Answer from the drawing. Dimensions are ordinates in mm from the lowest x, y and z of the part. Give positions to 0.01 mm unless a question says otherwise; leave off trailing zeros. Loops run counter-clockwise (first coordinate to the right, second up) from the corner with the lowest first, then second, coordinate; pieces in that order, holes last. Notation, with made-up numbers: (7, 40.25) -> (54, 40.25) arc R32 cw to (54, 72.25) -> close; hole circle Ø7 at (-38.5, 77.5). An arc over 180 degrees is marked (long way). Answer as CSV lines item,"result". Start each with the question number.
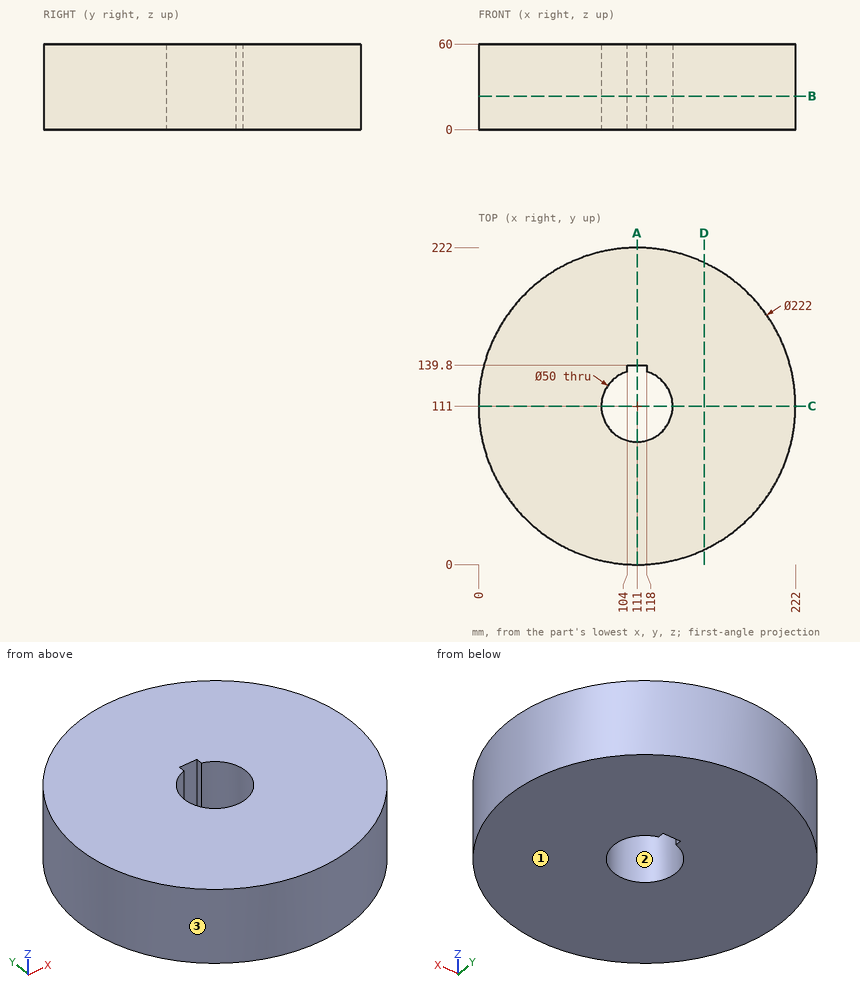
(1) Find section C-C on y = 111. Write down the section's boundary in (x, z), then the cut area to 3 significant figures.
(2) Each of these flat-tipped pins is pushed along its axis until it touches: P1, Ø5.5, axis at y = 136.5, z = 30, coming from the -X side; P2, Ø2.5, axis at y = 138, z = 20, coming from the +X side; P3, Ø10, axis at y = 53, z = 46.5, coming from the +X side. Where does it stop, or does it pass through?
(3) Find section B-B on z = 23.5. Write down the section's boundary in (x, y).
(4) Find the intervals of material crossed by line 1 along Y through (x, z) = (111, 36); line 2 along Y through (x, z) = (105.5, 41); line 3 along X through (y, z) = (127, 22), in increasing order. Write a range as from..to.
(5) The mould has two halves that part along Y. Classify the marked faces 1, 2 and 3: pulls with the +Y half, pulls with the -Y half, needs draft (parallel to the pull), parting line crosses it, or undercut.
(6) Find section A-A on x = 111. Write down the section's boundary in (y, z).
(7) Find section D-D on x = 158. Write down the section's boundary in (y, z), then the cut area to 3 significant figures.
Answer block:
1,outline,"(0, 0) -> (86, 0) -> (86, 60) -> (0, 60) -> close; (136, 0) -> (222, 0) -> (222, 60) -> (136, 60) -> close"
1,area,"10,300 mm2"
2,P1,"stops at x = 2.36"
2,P2,"stops at x = 218.97"
2,P3,"stops at x = 208.53"
3,outline,"circle Ø222 at (111, 111); hole (104, 135) arc R25 ccw (long way) to (118, 135) -> (118, 139.8) -> (104, 139.8) -> close"
4,line 1,"y = 0..86, 139.8..222"
4,line 2,"y = 0.14..86.61, 139.8..221.86"
4,line 3,"x = 1.16..91.79, 130.21..220.84"
5,face 1,"needs draft"
5,face 2,"undercut"
5,face 3,"parting line crosses it"
6,outline,"(0, 0) -> (86, 0) -> (86, 60) -> (0, 60) -> close; (139.8, 0) -> (222, 0) -> (222, 60) -> (139.8, 60) -> close"
7,outline,"(10.44, 0) -> (211.56, 0) -> (211.56, 60) -> (10.44, 60) -> close"
7,area,"12,100 mm2"
